Work out the finished part from the listing and answer in its coordinate system (mm). Face numbers are marked on the shaded views. A direction names the side the tool comes from. Coordinates: 2 decimals unless noted, no trailing zeros. Order: outer loops, then holes, each group sorted by start corner. A loop starts at its lowest first (then second) coordinate and runs counter-clockwise, first axis right, second up. Notation, with made-up numbers: M -12.5,68.5 L 12.5,68.5 A18 cw 12.5,99.5 Z; hole C -38.75,8 d5. An arc over 180 degrees is marked long. Use a Markdown table: item, result.
from build123d import *

# Parameters (mm, degrees)
BOSS_EXTRUDE1_DEPTH = 300
SKETCH3_R           = 112.5
SKETCH3_R_2         = 87.5
BOSS_EXTRUDE2_DEPTH = 170
SKETCH4_R           = 37.5
CUT_EXTRUDE1_DEPTH  = 170
SKETCH5_R           = 25
CUT_EXTRUDE2_DEPTH  = 170


with BuildPart() as part:
    # Sketch1 → Boss-Extrude1 (new body)
    with BuildSketch(Plane.XY):
        with BuildLine():
            Line((167.5, 0), (-167.5, 0))
            ThreePointArc((-167.5, 0), (-202.855339059, 14.644660941), (-217.5, 50))
            Line((-217.5, 50), (-217.5, 188))
            ThreePointArc((-217.5, 188), (-223.357864376, 202.142135624), (-237.5, 208))
            Line((-237.5, 208), (-475, 208))
            Line((-475, 208), (-475, 238))
            Line((-475, 238), (-237.5, 238))
            ThreePointArc((-237.5, 238), (-202.144660941, 223.355339059), (-187.5, 188))
            Line((-187.5, 188), (-187.5, 50))
            ThreePointArc((-187.5, 50), (-181.642135624, 35.857864376), (-167.5, 30))
            Line((-167.5, 30), (167.5, 30))
            ThreePointArc((167.5, 30), (181.642135624, 35.857864376), (187.5, 50))
            Line((187.5, 50), (187.5, 188))
            ThreePointArc((187.5, 188), (202.144660941, 223.355339059), (237.5, 238))
            Line((237.5, 238), (475, 238))
            Line((475, 238), (475, 208))
            Line((475, 208), (237.5, 208))
            ThreePointArc((237.5, 208), (223.357864376, 202.142135624), (217.5, 188))
            Line((217.5, 188), (217.5, 50))
            ThreePointArc((217.5, 50), (202.855339059, 14.644660941), (167.5, 0))
        make_face()
    extrude(amount=BOSS_EXTRUDE1_DEPTH)

    # Sketch3 → Boss-Extrude2 (add)
    with BuildSketch(Plane(origin=(0, 30, 0), x_dir=(1, 0, 0), z_dir=(0, 1, 0))):
        with Locations((0, -150)):
            Circle(SKETCH3_R)
        with Locations((0, -150)):
            Circle(SKETCH3_R_2, mode=Mode.SUBTRACT)
    extrude(amount=BOSS_EXTRUDE2_DEPTH)

    # Sketch4 → Cut-Extrude1 (cut)
    with BuildSketch(Plane(origin=(0, 30, 0), x_dir=(1, 0, 0), z_dir=(0, 1, 0))):
        with Locations((0, -150)):
            Circle(SKETCH4_R)
    extrude(amount=-CUT_EXTRUDE1_DEPTH, mode=Mode.SUBTRACT)

    # Sketch5 → Cut-Extrude2 (cut)
    with BuildSketch(Plane(origin=(0, 238, 0), x_dir=(1, 0, 0), z_dir=(0, 1, 0))):
        with Locations((355, -150)):
            Circle(SKETCH5_R)
        with Locations((-355, -150)):
            Circle(SKETCH5_R)
    extrude(amount=-CUT_EXTRUDE2_DEPTH, mode=Mode.SUBTRACT)


solid = part.part
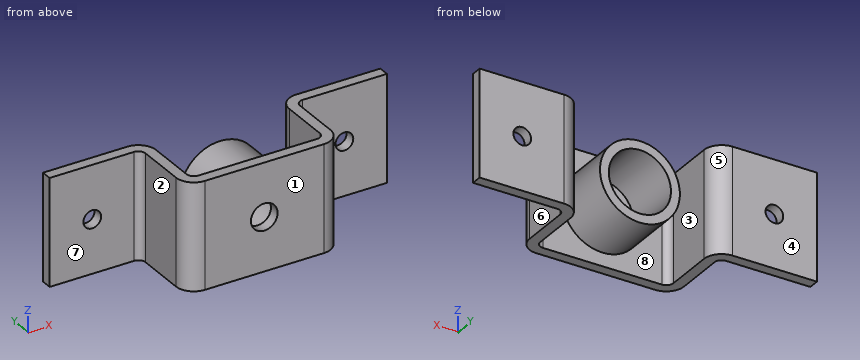
1. For a pull along X with two mould halves and no side action, classify the marked faces 1, 2 and 3 as +X half, -X half, draft (parallel to the pull), parting line (faces both ways), or undercut.
Answers below:
| item | result |
|---|---|
| face 1 | draft |
| face 2 | -X half |
| face 3 | undercut |
2. Section C-C on z = 215.5 is taken. Determine the outline of the cut face in (x, y), then the cut area to 4 significant figures.
Answers below:
| item | result |
|---|---|
| outline | M -475,208 L -237.5,208 A20 cw -217.5,188 L -217.5,50 A50 ccw -167.5,0 L 167.5,0 A50 ccw 217.5,50 L 217.5,188 A20 cw 237.5,208 L 475,208 L 475,238 L 237.5,238 A50 ccw 187.5,188 L 187.5,50 A20 cw 167.5,30 L 91.47,30 L 91.47,200 L 58.02,200 L 58.02,30 L -58.02,30 L -58.02,200 L -91.47,200 L -91.47,30 L -167.5,30 A20 cw -187.5,50 L -187.5,188 A50 ccw -237.5,238 L -475,238 Z |
| area | 50,550 mm² |
3. Section D-D on z = 139.5 is taken. Give the number of separate pieces and of enclosed holes in the cut face, then the cut area to 3 significant figures.
Answers below:
| item | result |
|---|---|
| separate pieces | 4 |
| enclosed holes | 0 |
| area | 42,800 mm² |
4. For the marked faces 4, 5, 6, 7 and 8, determine the directions among +Z, -Z, +X, -X, +Y, -Y from which every point of the face is accessible in a straight line to the end or side of a thin tool.
Answers below:
| item | result |
|---|---|
| face 4 | +Z, -Z, +X, -X, +Y |
| face 5 | +Z, -Z, +Y |
| face 6 | +Z, -Z, +X, -Y |
| face 7 | +Z, -Z, -X, -Y |
| face 8 | +Y |
5. Find the intervals of material crossed by probe 1 along X at (y, z) = (93, 27.5); probe 2 along X at (y, z) = (46, 184); probe 3 along Z at (x, y) = (-355, 221), in increasing order.
Answers below:
| item | result |
|---|---|
| probe 1 | -217.5 to -187.5, 187.5 to 217.5 |
| probe 2 | -217.34 to -187.1, -107.24 to -80.62, 80.62 to 107.24, 187.1 to 217.34 |
| probe 3 | 0 to 125, 175 to 300 |
6. Section A-A on y = 62 is taken. Determine the outline of the cut face in (x, z).
Answers below:
| item | result |
|---|---|
| outline | M -217.5,0 L -187.5,0 L -187.5,300 L -217.5,300 Z; C 0,150 d225; M 187.5,0 L 217.5,0 L 217.5,300 L 187.5,300 Z; hole C 0,150 d175 |
7. Section B-B on x = 355 is taken. Determine the outline of the cut face in (y, z).
Answers below:
| item | result |
|---|---|
| outline | M 208,0 L 238,0 L 238,125 L 208,125 Z; M 208,175 L 238,175 L 238,300 L 208,300 Z |
8. Flat-ended cylindrical pins translate along their axes: P1, Ø6, axis at x = -315, z = 178, coming from the -Y side; P2, Ø8, axis at x = 50.5, z = 136, coming from the +Y side; P3, Ø6, axis at x = 54, y = 156.5, coming from the +Z side. Find the tip coordinate at first contact, or state that the pin passes through.
Answers below:
| item | result |
|---|---|
| P1 | y = 208 |
| P2 | y = 30 |
| P3 | z = 250.28 |
